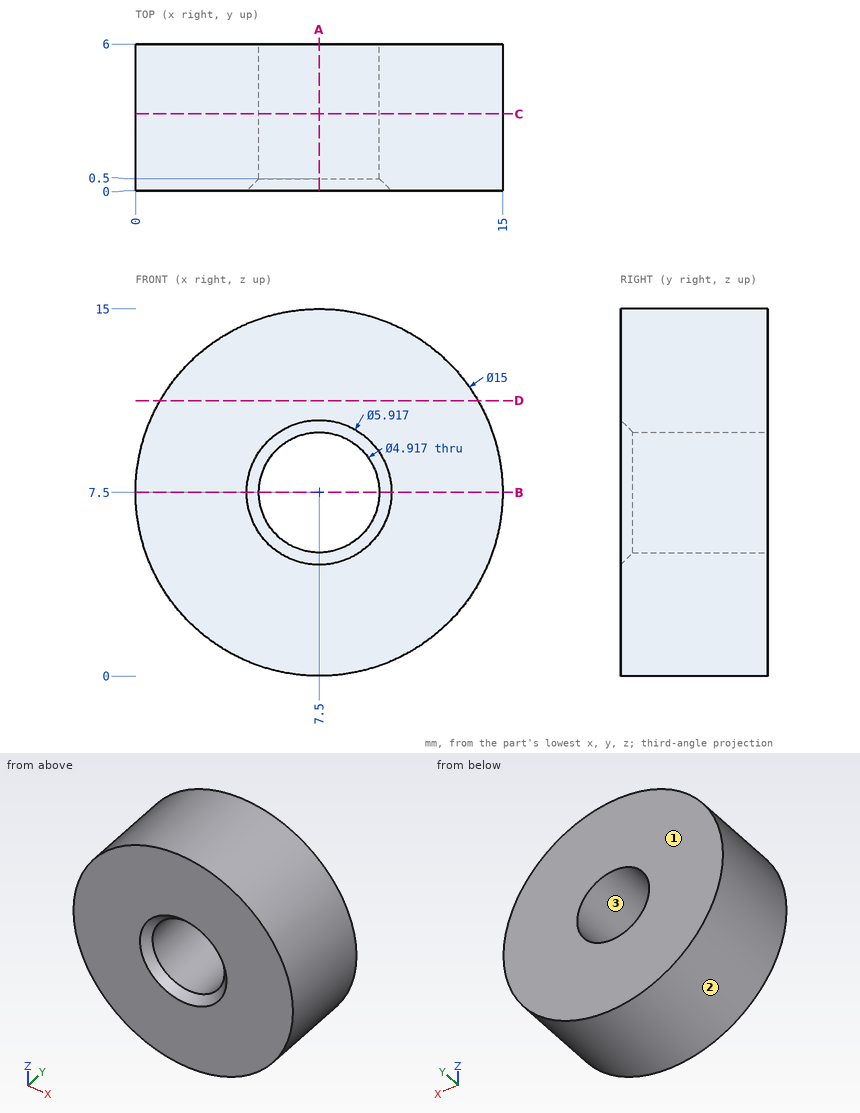
Source: three-view drawing plus pictorial views. Frame: mm from the lowest corner of the part. Coordinates: 2 decimals unless noted, no trailing zeros. Write each loop counter-clockwise with the first axis right and the second up, starting at its lowest first coordinate (ties: lowest second). Pieces come first, ordered by that corner, then holes. Notation, with made-up numbers: (67, 47.25) - (78, 47.25) arc R13 cw to (78, 59.25) - close; hole circle Ø11 at (-35.5, 58). An arc over 180 degrees is marked (long way). Return JSON: item names as keys, results as strings.
Item 1: Line query: L1, parallel to Z at x = 7.5, y = 4.2; L2, parallel to Z at x = 9, y = 1.2; L3, parallel to X at y = 4.15, z = 5.75. Output: solid intervals per line, ascending.
Completed:
{"L1": "z = 0 to 5.04, 9.96 to 15", "L2": "z = 0.15 to 5.55, 9.45 to 14.85", "L3": "x = 0.21 to 5.77, 9.23 to 14.79"}
Item 2: Pull-direction query (Z, two-part tool) for the marked faces 1, 2 and 3; classes: +Z half, -Z half, draft (parallel to the pull), parting line (faces both ways), or undercut.
Completed:
{"face 1": "draft", "face 2": "parting line", "face 3": "undercut"}
Item 3: Section query C-C (y = 3.15). Output: boundary loops of the cut face in (x, z), and give its area (3 significant figures).
Completed:
{"outline": "circle Ø15 at (7.5, 7.5); hole circle Ø4.92 at (7.5, 7.5)", "area": "158 mm2"}
Item 4: Pin query (flat end, axial travel): pin 1 Ø1.5 at (x, y) = (11, 4.5) entering from +Z; pin 2 Ø2 at (x, y) = (5.5, 5) entering from -Z; pin 3 Ø1.5 at (x, y) = (2, 5) entering from +Z. Return the tip coordinate at first contact, or that it passes through.
Completed:
{"pin 1": "stops at z = 14.48", "pin 2": "stops at z = 0.07", "pin 3": "stops at z = 13.3"}
Item 5: Section query A-A (x = 7.5). Output: boundary loops of the cut face in (y, z).
Completed:
{"outline": "(0, 0) - (6, 0) - (6, 5.04) - (0.5, 5.04) - (0, 4.54) - close; (0, 10.46) - (0.5, 9.96) - (6, 9.96) - (6, 15) - (0, 15) - close"}
Item 6: Section query B-B (z = 7.5). Output: boundary loops of the cut face in (x, y), and give its area (3 significant figures).
Completed:
{"outline": "(0, 0) - (4.54, 0) - (5.04, 0.5) - (5.04, 6) - (0, 6) - close; (9.96, 0.5) - (10.46, 0) - (15, 0) - (15, 6) - (9.96, 6) - close", "area": "60.2 mm2"}
Item 7: Section query D-D (z = 11.25). Output: boundary loops of the cut face in (x, y).
Completed:
{"outline": "(1, 0) - (14, 0) - (14, 6) - (1, 6) - close"}
